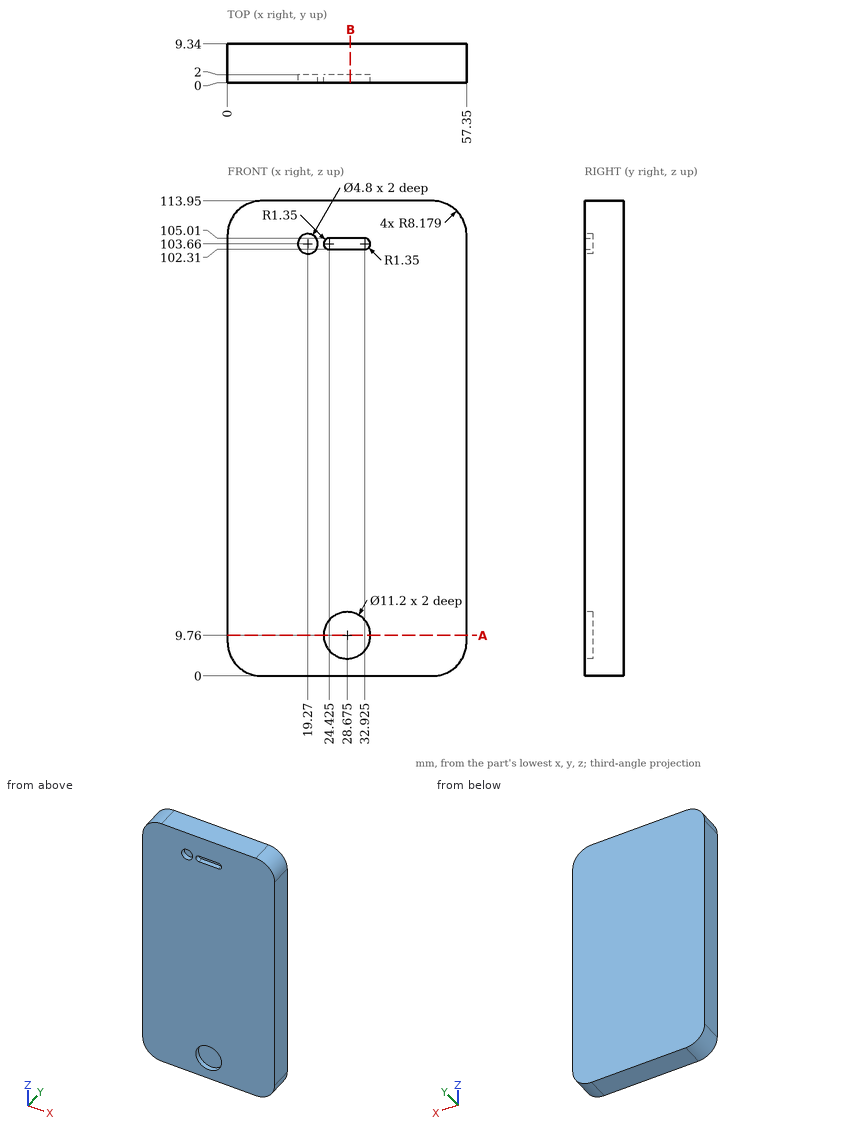
Geometry check sheet. Reference: drawing and pictorial views, mm from the part's lowest x, y, z. Give positions to 0.01 mm unless a question says otherwise; leave off trailing zeros. Order: outer loops, then holes, each group sorted by start corner. A loop starts at its lowest first (then second) coordinate and runs counter-clockwise, first axis right, second up. Notation, with made-up numbers: M -15,23.25 L 35,23.25 A18 ccw 35,28.25 Z; hole C 29,57 d1. An arc over 180 degrees is marked long. Answer in a Markdown table with one row per item. Add a question column.
Q1. Thickness scan on L1, parallel to Z at x = 19.27, y = 1.6; L2, parallel to X at y = 4, z = 8; L3, parallel to Y at x = 31, z = 104. Record the ranges inside material, lowest first.
Q2. Sectioned sample at B-B, the plane x = 29.5. Record the boundary of the cut face in (y, z), and give its area (3 significant figures).
Q3. Sectioned sample at A-A, the plane z = 9.76. Record the boundary of the cut face in (x, y) (3 decimals), and give its area (3 significant figures).
Q4. Gauge pin test, flat end, axial feed: pin 1 Ø4 at (x, z) = (19.27, 103.66) entering from -Y. Record the tip position at first contact, or that the pin passes through.
Verdict:
| question | item | result |
|---|---|---|
| 1 | L1 | 0 to 101.26, 106.06 to 113.95 |
| 1 | L2 | 0 to 57.35 |
| 1 | L3 | 2 to 9.34 |
| 2 | outline | M 0,0 L 9.34,0 L 9.34,113.95 L 0,113.95 L 0,105.01 L 2,105.01 L 2,102.31 L 0,102.31 L 0,15.3 L 2,15.3 L 2,4.22 L 0,4.22 Z |
| 2 | area | 1,040 mm² |
| 3 | outline | M 0,0 L 23.075,0 L 23.075,2 L 34.275,2 L 34.275,0 L 57.35,0 L 57.35,9.34 L 0,9.34 Z |
| 3 | area | 513 mm² |
| 4 | pin 1 | y = 2 |
